Autodesk Inventor part; units mm, degrees
ref_plane "YZ Plane" through (0, 0, 0) normal (1, 0, 0) x (0, 1, 0)
ref_plane "XZ Plane" through (0, 0, 0) normal (0, 1, 0) x (-1, 0, 0)
ref_plane "XY Plane" through (0, 0, 0) normal (0, 0, 1) x (1, 0, 0)
ref_plane "Płaszczyzna konstrukcyjna1" through (0, 0, 0) normal (0, 0, 1) x (1, 0, 0)
sketch "Szkic1" plane through (0, 0, 0) normal (0, 0, 1) x (1, 0, 0)
  line L0 (60.3592, 11) -> (60.3592, -11)
  line L1 (70.3592, 11) -> (70.3592, -11)
  line L2 (70.3592, -11) -> (60.3592, -11)
  line L3 (60.3592, -11) -> (60.3592, 11)
  line L4 (60.3592, 11) -> (70.3592, 11)
  line L5 (70.3592, 11) -> (70.3592, -11)
  point P0 (0, 0)
extrude "Wyciągnięcie proste1" add sketch "Szkic1" along normal blind 76
sketch "Szkic2" plane through (0, 0, 0) normal (0, 0, -1) x (-1, 0, 0)
  circle A0 centre (-65.3592, 0) radius 2.125
  line L0 (-70.3592, 11) -> (-60.3592, 11) construction
  line L1 (-65.3592, 0) -> (-70.3592, 11) construction
  line L2 (-60.3592, 11) -> (-65.3592, 0) construction
  line L3 (-60.3592, 11) -> (-60.3592, -11) construction
  line L4 (-65.3592, 0) -> (-60.3592, -11) construction
  point P0 (0, 0)
  dimension "d13" = 4.25
extrude "Wyciągnięcie proste3" cut sketch "Szkic2" against normal through all
sketch "Szkic4" plane through (60.3592, -11, 0) normal (-1, 0, 0) x (0, 0, 1)
  line L0 (0, 22) -> (0, 0)
  line L1 (0, 0) -> (76, 0)
  line L2 (76, 22) -> (76, 0)
  line L3 (0, 22) -> (76, 22)
  line L4 (68, 7.375) -> (64.55, 7.375)
  line L5 (64.55, 7.375) -> (64.55, 14.625)
  line L6 (64.55, 14.625) -> (68, 14.625)
  line L7 (68, 14.625) -> (68, 7.375)
  line L8 (11.45, 7.375) -> (8, 7.375)
  line L9 (8, 7.375) -> (8, 14.625)
  line L10 (8, 14.625) -> (11.45, 14.625)
  line L11 (11.45, 14.625) -> (11.45, 7.375)
  line L12 (0, 0) -> (76, 0)
  line L13 (76, 0) -> (68, 7.375) construction
  line L14 (68, 14.625) -> (76, 22) construction
  point P0 (0, 11)
  dimension "d14" = 7.25
  dimension "d15" = 3.45
  dimension "d16" = 3.45
  dimension "d17" = 8
  dimension "d18" = 8
extrude "Wyciągnięcie proste4" cut sketch "Szkic4" against normal blind 8.5 contours L4 L5 L6 L7 | L8 L9 L10 L11
sketch "Szkic3" plane through (70.3592, -11, 0) normal (1, 0, 0) x (0, 0, -1)
  line L0 (-66, 15) -> (-62.5, 15)
  line L1 (-62.5, 15) -> (-62.5, 7)
  line L2 (-62.5, 7) -> (-66, 7)
  line L3 (-66, 7) -> (-66, 15)
  line L4 (-13.5, 15) -> (-10, 15)
  line L5 (-10, 15) -> (-10, 7)
  line L6 (-10, 7) -> (-13.5, 7)
  line L7 (-13.5, 7) -> (-13.5, 15)
  line L8 (0, 22) -> (-76, 22)
  line L9 (0, 0) -> (-76, 0)
  line L10 (-76, 0) -> (-76, 22)
  line L11 (0, 0) -> (0, 22)
  line L12 (-66, 22) -> (-66, 15) construction
  line L13 (-66, 0) -> (-66, 7) construction
  point P0 (0, 11)
  dimension "d2" = 10
  dimension "d3" = 10
  dimension "d4" = 3.5
  dimension "d6" = 8
  dimension "d7" = 3.5
equation "\"d16\" = d15"
equation "\"d18\" = d17"
equation "\"d3\" = d2"
equation "\"d7\" = d4"
properties part number "coupler"
The listing builds one solid part. Answer for the finished solid, in the listing's coordinates (mm). A direction names the side the tool comes from. Give positions to 0.01 mm unless a question says otherwise; leave off trailing zeros. Order: outer loops, then holes, each group sorted by start corner. A loop starts at its lowest first (then second) coordinate and runs counter-clockwise, first axis right, second up. Notation, with made-up numbers: (-22.75, -21.75) - (-13.75, -21.75) arc R26 cw to (-13.75, -2.75) - close; hole circle Ø2 at (-6, 54.25). An arc over 180 degrees is marked (long way). Use one line per item in the form item = value. Start each with the question number.
(1) Consider line 1 (Z direction, x = 62.25, y = 2.5); line 2 (Y direction, x = 62.25, z = 10) (3 decimals); line 3 (Y direction, x = 65.5, z = 69). Determine where each line is inside the solid, lowest interval first. Write a range as from..to.
(2) A cutting plane is placed at B-B, the plane x = 64.75. Write down the section's boundary in (y, z) (3 decimals), then the cut area to 3 significant figures.
(3) A flat-ended cylindrical pin translates along its axis: pin 1 Ø1 at (y, z) = (1.5, 66.5) entering from -X. Find the tip coordinate at first contact, or state that the pin passes through.
(4) The mould has two halves that part along Z. Classify faces 3 (the flat face through (68, 0, 76)), 4 (the flat face through (65, -3.625, 10)), 5 (the flat face through (70.359, 0, 37)), 6 (the flat face through (65, -3.625, 66)): released by +Z, released by -Z, zero draft, split by the parting line, or undercut.
(5) For faces 1 (the cylindrical face through (67.482, 0.093, 37.628)), 2 (the flat face through (68.859, 0, 66)), determine the directions among +Z, -Z, +X, -X, +Y, -Y from which every point of the face is accessible in a straight line to the end or side of a thin tool.
(6) A cutting plane is placed at A-A, the plane y = 0. Write down the section's boundary in (x, z).
(7) A cutting plane is placed at C-C, the plane z = 61.5. Write down the section's boundary in (x, y) (3 decimals).
Ans:
q1.line_1 = 0..8, 11.45..64.55, 68..76
q1.line_2 = -11..-3.625, 3.625..11
q1.line_3 = -11..-2.12, 2.12..11
q2.outline = (-11, 0) - (-2.036, 0) - (-2.036, 8) - (-3.625, 8) - (-3.625, 11.45) - (-2.036, 11.45) - (-2.036, 64.55) - (-3.625, 64.55) - (-3.625, 68) - (-2.036, 68) - (-2.036, 76) - (-11, 76) - close; (2.036, 0) - (11, 0) - (11, 76) - (2.036, 76) - (2.036, 68) - (3.625, 68) - (3.625, 64.55) - (2.036, 64.55) - (2.036, 11.45) - (3.625, 11.45) - (3.625, 8) - (2.036, 8) - close
q2.area = 1,340 mm^2
q3.pin_1 = 68.86
q4.face_3 = released by +Z
q4.face_4 = undercut
q4.face_5 = zero draft
q4.face_6 = undercut
q5.face_1 = +Z, -Z
q5.face_2 = -X
q6.outline = (60.36, 0) - (63.23, 0) - (63.23, 8) - (60.36, 8) - close; (60.36, 11.45) - (63.23, 11.45) - (63.23, 64.55) - (60.36, 64.55) - close; (60.36, 68) - (63.23, 68) - (63.23, 76) - (60.36, 76) - close; (67.48, 0) - (70.36, 0) - (70.36, 76) - (67.48, 76) - (67.48, 68) - (68.86, 68) - (68.86, 64.55) - (67.48, 64.55) - (67.48, 11.45) - (68.86, 11.45) - (68.86, 8) - (67.48, 8) - close
q7.outline = (60.359, -11) - (70.359, -11) - (70.359, 11) - (60.359, 11) - close; hole circle Ø4.25 at (65.359, 0)
